Work out the finished part from the listing and answer in its coordinate system (mm). Face numbers are marked on the shaded views. A direction names the side the tool comes from. Coordinates: 2 decimals unless noted, no trailing zeros. Write each loop counter-clockwise with the first axis right and the second up, starting at its lowest first coordinate (ties: lowest second). Pieces come first, ordered by that corner, then holes. Notation, with made-up numbers: (66.5, 32) - (98.5, 32) arc R11 cw to (98.5, 50) - close; hole circle Ø9 at (35, 72). An arc over 180 degrees is marked (long way). Use a Markdown table: item, result. Add a question column.
(1) The part is cut by section A-A, the plane y = -105.41. Give the vertices of the cut face in (x, z).
(2) Find the intervals of material crossed by line 1 (Y direction, x = -96, z = 7); line 2 (Z direction, x = -115.5, y = -93), in increasing order. Write a range as from..to.
(3) The part is cut by section D-D, the plane y = -54. Give the vertices of the cut face in (x, z), then the cut area to 3 significant figures.
(4) A tool of negligible diameter and unlimited length cuts with its end or side. For the marked faces 1 and 2, from which of +Z, -Z, +X, -X, +Y, -Y can it reach the whole face along a straight path? Write none if from no direction.
(5) Given pin 1 Ø12 at (x, y) = (-70, -46) entering from -Z; pin 2 Ø12 at (y, z) = (-105.41, -96.52) entering from -X, each flat-ended and moving along its own axis, determine where each tip first touches the part or whether it passes through.
(6) The part is cut by section C-C, the plane x = -96.52. Give the vertices of the cut face in (y, z), then the cut area to 3 significant figures.
(7) The part is cut by section B-B, the plane z = -96.52. Give the vertices of the cut face in (x, y).
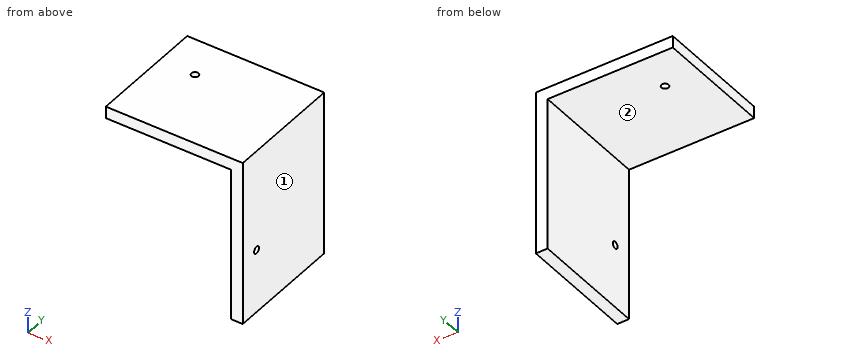
from build123d import *

# Parameters (mm, degrees)
F1_DEPTH = 127
F2_R     = 3.81
F3_DEPTH = 25.4
F4_R     = 3.81
F5_DEPTH = 25.4


with BuildPart() as f1:
    # F0 (on Front) → F1 (new body)
    with BuildSketch(Plane.XZ):
        Polygon((-134.62, 0), (0, 0), (0, -165.1), (12.7, -165.1), (12.7, 12.7), (-134.62, 12.7), align=None)
    extrude(amount=F1_DEPTH)

    # F2 (on face) → F3 (cut)
    with BuildSketch(Plane(origin=(0, 0, 0), x_dir=(1, 0, 0), z_dir=(0, 0, -1))):
        with Locations((-96.52, 43.188728)):
            Circle(F2_R)
    extrude(amount=-F3_DEPTH, mode=Mode.SUBTRACT)

    # F4 (on face) → F5 (cut)
    with BuildSketch(Plane(origin=(0, 0, 0), x_dir=(0, -1, 0), z_dir=(-1, 0, 0))):
        with Locations((105.41, -96.52)):
            Circle(F4_R)
    extrude(amount=-F5_DEPTH, mode=Mode.SUBTRACT)


solid = f1.part
Model answer:
| question | item | result |
|---|---|---|
| 1 | outline | (-134.62, 0) - (0, 0) - (0, -92.71) - (12.7, -92.71) - (12.7, 12.7) - (-134.62, 12.7) - close; (0, -165.1) - (12.7, -165.1) - (12.7, -100.33) - (0, -100.33) - close |
| 2 | line 1 | -127..-46.96, -39.41..0 |
| 2 | line 2 | 0..12.7 |
| 3 | outline | (-134.62, 0) - (0, 0) - (0, -165.1) - (12.7, -165.1) - (12.7, 12.7) - (-134.62, 12.7) - close |
| 3 | area | 3,970 mm^2 |
| 4 | face 1 | +Z, -Z, +X, +Y, -Y |
| 4 | face 2 | -Z, -X, +Y, -Y |
| 5 | pin 1 | z = 0 |
| 5 | pin 2 | x = 0 |
| 6 | outline | (-127, 0) - (-47, 0) - (-47, 12.7) - (-127, 12.7) - close; (-39.38, 0) - (0, 0) - (0, 12.7) - (-39.38, 12.7) - close |
| 6 | area | 1,520 mm^2 |
| 7 | outline | (0, -127) - (12.7, -127) - (12.7, -109.22) - (0, -109.22) - close; (0, -101.6) - (12.7, -101.6) - (12.7, 0) - (0, 0) - close |
